Model file for the job. Use its own axes, mm. A direction names the side the tool comes from. Round coordinates to 2 decimals unless told otherwise and drop trailing zeros. Write each loop counter-clockwise with the first axis right and the second up, starting at its lowest first coordinate (ties: lowest second). Pieces come first, ordered by that corner, then holes. Notation, with made-up numbers: (35.25, 45.5) - (66.25, 45.5) arc R23 cw to (66.25, 58.5) - close; hole circle Ø1 at (49, 0). An arc over 180 degrees is marked (long way). Answer as a JSON object with one key per item and string values. Group by question number.
from build123d import *

# Parameters (mm, degrees)
SKETCH_2_W      = 40
SKETCH_2_H      = 56
EXTRUDE_1_DEPTH = 20
SKETCH_3_R      = 8.41555303
SKETCH_3_R_2    = 6.928356998
EXTRUDE_2_DEPTH = 10
FILLET_1_R      = 5


with BuildPart() as part:
    # 草图2 → 凸台-拉伸1 (new body)
    with BuildSketch(Plane(origin=(0, 0, 0), x_dir=(1, 0, 0), z_dir=(0, 1, 0))):
        Rectangle(SKETCH_2_W, SKETCH_2_H)
    extrude(amount=EXTRUDE_1_DEPTH)

    # 草图3 → 凸台-拉伸2 (add)
    with BuildSketch(Plane.XY.offset(28)):
        with Locations(Location((0, 10, 0), (0, 0, 180))):
            Circle(SKETCH_3_R)
        with Locations((0, 10)):
            Circle(SKETCH_3_R_2, mode=Mode.SUBTRACT)
    extrude(amount=EXTRUDE_2_DEPTH)

    # 圆角1
    fillet_1_edges = [part.edges().sort_by_distance(p)[0] for p in [
        (20, 10, 28),
        (-20, 10, 28),
        (-20, 10, -28),
        (20, 10, -28),
    ]]
    fillet(fillet_1_edges, radius=FILLET_1_R)


solid = part.part
(1) Slice it at D-D (y = 5). Write the cut outline in (x, z).
(2) Slice it at A-A (x = 0). Write the cut outline in (y, z), then the cut area to 3 significant figures.
(3) Drill centre lines: line 1 (Y direction, x = 0, z = 35.75); line 2 (Z direction, x = 8.5, y = 17); line 3 (Z direction, x = -17, y = 10.75). Where is each one in solid material? Low to high. Write a range as from..to.
(4) 3-axis set-ups, long thin cutter, end or side, ignore diameter. For faces 1 (the flat face through (-20, 10, 0)), 2 (the flat face through (0, 1, 28)): which of +Z, -Z, +X, -X, +Y, -Y reach the whole face in a straight line?
(5) Slice it at B-B (z = 31). Write the cut outline in (x, y).
(6) Pull direction Y, two halves, no side cores. Call faces 3 (the cylindrical face through (-1.502, 3.236, 32.93)), 4 (the flat face through (0, 10, 28)), 5 (the cylindrical face through (-19, 10, 26)), 6 (the flat face through (0, 20, 0)): pulls with the +Y half, pulls with the -Y half, needs draft (parallel to the pull), parting line crosses it, or undercut.
(7) Slice it at C-C (y = 10). Write the cut outline in (x, z), then the cut area to 3 significant figures.
Answer:
{
 "1": {"outline": "(-20, -23) arc R5 ccw to (-15, -28) - (15, -28) arc R5 ccw to (20, -23) - (20, 23) arc R5 ccw to (15, 28) - (6.77, 28) - (6.77, 38) - (4.8, 38) - (4.8, 28) - (-4.8, 28) - (-4.8, 38) - (-6.77, 38) - (-6.77, 28) - (-15, 28) arc R5 ccw to (-20, 23) - close"},
 "2": {"outline": "(0, -28) - (20, -28) - (20, 28) - (18.42, 28) - (18.42, 38) - (16.93, 38) - (16.93, 28) - (3.07, 28) - (3.07, 38) - (1.58, 38) - (1.58, 28) - (0, 28) - close", "area": "1,150 mm²"},
 "3": {"line 1": "1.58..3.07, 16.93..18.42", "line 2": "-28..28", "line 3": "-27.58..27.58"},
 "4": {"face 1": "+Z, -Z, -X, +Y, -Y", "face 2": "+Z"},
 "5": {"outline": "circle Ø16.83 at (0, 10); hole circle Ø13.86 at (0, 10)"},
 "6": {"face 3": "undercut", "face 4": "undercut", "face 5": "needs draft", "face 6": "pulls with the +Y half"},
 "7": {"outline": "(-20, -23) arc R5 ccw to (-15, -28) - (15, -28) arc R5 ccw to (20, -23) - (20, 23) arc R5 ccw to (15, 28) - (8.42, 28) - (8.42, 38) - (6.93, 38) - (6.93, 28) - (-6.93, 28) - (-6.93, 38) - (-8.42, 38) - (-8.42, 28) - (-15, 28) arc R5 ccw to (-20, 23) - close", "area": "2,250 mm²"}
}
